Source: CAD feature listing. Evaluate the final solid. Frame: model axes, mm. Face numbers are marked on the shaded views. A direction names the side the tool comes from. Coordinates: 2 decimals unless noted, no trailing zeros. Order: outer loops, then holes, each group sorted by start corner. A loop starts at its lowest first (then second) coordinate and runs counter-clockwise, first axis right, second up. Notation, with made-up numbers: (37.25, 67.5) - (75.25, 67.5) arc R19 cw to (75.25, 94.5) - close; hole circle Ø9 at (4.25, 52). An arc over 180 degrees is marked (long way). One line per question, with ' | ' between items. Start each with the question number.
(1) Draft query along Z for the marked faces 1, 2, 3 and 4. Return one class per face: +Z half, -Z half, draft (parallel to the pull), parting line (faces both ways), or undercut.
(2) Section A-A (y = 4.75). Return the cut outline in (x, z), then the cut area to 3 significant figures.
(3) Contact query for flat-ended pins moving along their axis: P1, Ø5.5, axis at x = 0, z = 0, coming from the -Y side; P2, Ø4, axis at y = 17, z = -0.5, coming from the +X side; P3, Ø5, axis at x = -3, y = 21, coming from the +Z side. Output: stop coordinate, or through.
(4) Section B-B (z = 0). Return the cut outline in (x, y), then the cut area to 3 significant figures.
(5) Section D-D (x = -1.75). Return the cut outline in (y, z).
(6) Access query for the marked faces 5 and 6. Directions: +Z, -Z, +X, -X, +Y, -Y. A direction counts if a zero-diameter tool reaches every point of the face in a straight line with its end or side. Return the directions, or none.
(7) Section C-C (x = -0.5). Return the cut outline in (y, z).
(8) Line query: line 1 along X through (y, z) = (6, 0); line 2 along Z through (x, y) = (0.5, 18); line 3 along Z through (x, y) = (0.5, 3.25). Output: solid intervals per line, ascending.
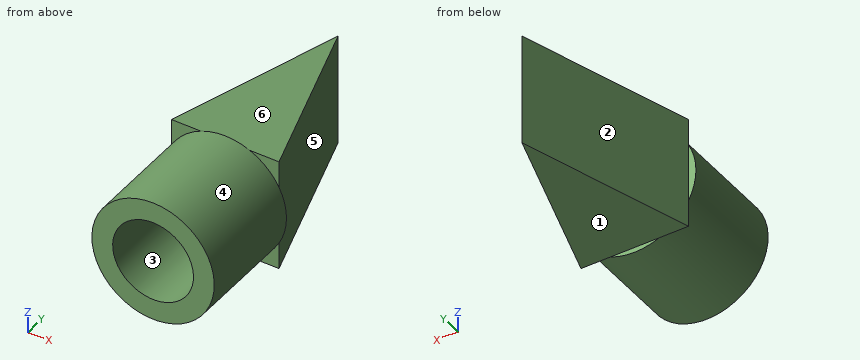
from build123d import *

# Parameters (mm, degrees)
SKETCH1_R           = 5.3
SKETCH1_R_2         = 3.5
BOSS_EXTRUDE1_DEPTH = 9.6
BOSS_EXTRUDE2_DEPTH = 4.86


with BuildPart() as part:
    # Sketch1 → Boss-Extrude1 (new body)
    with BuildSketch(Plane(origin=(0, 0, 0), x_dir=(1, 0, 0), z_dir=(0, 1, 0))):
        with Locations(Location((0, 0, 0), (0, 0, 270))):
            Circle(SKETCH1_R)
        with Locations(Location((0, 0, 0), (0, 0, 270))):
            Circle(SKETCH1_R_2, mode=Mode.SUBTRACT)
    extrude(amount=BOSS_EXTRUDE1_DEPTH)

    # Sketch2 → Boss-Extrude2 (add, symmetric)
    with BuildSketch(Plane.XY):
        Polygon((-4.65, 9.6), (4.65, 9.6), (0, 24.6), align=None)
    extrude(amount=BOSS_EXTRUDE2_DEPTH, both=True)


solid = part.part
Response values:
1) face 1: -Z half | face 2: draft | face 3: undercut | face 4: parting line
2) outline: circle Ø10.6 at (0, 0); hole circle Ø7 at (0, 0) | area: 49.8 mm²
3) P1: stops at y = 9.6 | P2: stops at x = 2.98 | P3: stops at z = 4.86
4) outline: (-5.3, 0) - (-3.5, 0) - (-3.5, 9.6) - (3.5, 9.6) - (3.5, 0) - (5.3, 0) - (5.3, 9.6) - (4.65, 9.6) - (0, 24.6) - (-4.65, 9.6) - (-5.3, 9.6) - close | area: 104 mm²
5) outline: (0, -5) - (9.6, -5) - (9.6, -4.86) - (18.95, -4.86) - (18.95, 4.86) - (9.6, 4.86) - (9.6, 5) - (0, 5) - (0, 3.03) - (9.6, 3.03) - (9.6, -3.03) - (0, -3.03) - close
6) face 5: +Z, -Z, +X, +Y | face 6: +Z, +X, -X, +Y
7) outline: (0, -5.28) - (9.6, -5.28) - (9.6, -4.86) - (22.99, -4.86) - (22.99, 4.86) - (9.6, 4.86) - (9.6, 5.28) - (0, 5.28) - (0, 3.46) - (9.6, 3.46) - (9.6, -3.46) - (0, -3.46) - close
8) line 1: x = -5.3 to -3.5, 3.5 to 5.3 | line 2: z = -4.86 to 4.86 | line 3: z = -5.28 to -3.46, 3.46 to 5.28
